Design review of the part built by this model. Coordinates are the model's own, in mm. Give positions to 0.01 mm unless a question says otherwise; leave off trailing zeros. Loops run counter-clockwise (first coordinate to the right, second up) from the corner with the lowest first, then second, coordinate; pieces in that order, holes last. Notation, with made-up numbers: (86.25, -24) - (106.25, -24) arc R11 ccw to (106.25, -6) - close; hole circle Ø11 at (-16.75, 32.25). An arc over 180 degrees is marked (long way). Write each question's results on one line, items separated by ' | '.
```python
from build123d import *

# Parameters (mm, degrees)
SKETCH1_W           = 279.4
SKETCH1_H           = 311.15
SKETCH1_W_2         = 114.3
SKETCH1_H_2         = 12.7
SKETCH1_W_3         = 12.7
SKETCH1_H_3         = 114.3
BOSS_EXTRUDE1_DEPTH = 3.3528
SKETCH2_R           = 9.525
CUT_EXTRUDE1_DEPTH  = 6.7056


with BuildPart() as part:
    # Sketch1 → Boss-Extrude1 (new body)
    with BuildSketch(Plane.XY):
        Rectangle(SKETCH1_W, SKETCH1_H)
        with Locations((-73.025, -161.925)):
            Rectangle(SKETCH1_W_2, SKETCH1_H_2)
        with Locations((73.025, -161.925)):
            Rectangle(SKETCH1_W_2, SKETCH1_H_2)
        with Locations((-146.05, -70.64375)):
            Rectangle(SKETCH1_W_3, SKETCH1_H_3)
        with Locations((-146.05, 70.64375)):
            Rectangle(SKETCH1_W_3, SKETCH1_H_3)
        with Locations((73.025, 161.925)):
            Rectangle(SKETCH1_W_2, SKETCH1_H_2)
        with Locations((-73.025, 161.925)):
            Rectangle(SKETCH1_W_2, SKETCH1_H_2)
    extrude(amount=BOSS_EXTRUDE1_DEPTH)

    # Sketch2 → Cut-Extrude1 (cut)
    with BuildSketch(Plane.XY.offset(3.3528)):
        with Locations((117.475, 69.85)):
            Circle(SKETCH2_R)
        with Locations((117.475, -69.85)):
            Circle(SKETCH2_R)
    extrude(amount=-CUT_EXTRUDE1_DEPTH, mode=Mode.SUBTRACT)


solid = part.part
```
Item 1: Wall thickness on probe 1 along Y at (x, z) = (118, 2.05) (3 decimals): over which ranges is the line inside the solid? List them lowest first.
Output values:
probe 1: y = -168.275 to -79.361, -60.339 to 60.339, 79.361 to 168.275
Item 2: We need section A-A on y = 69.85. Give the boundary of the cut face in (x, z), then the cut area to 3 significant figures.
Output values:
outline: (-152.4, 0) - (107.95, 0) - (107.95, 3.35) - (-152.4, 3.35) - close; (127, 0) - (139.7, 0) - (139.7, 3.35) - (127, 3.35) - close | area: 915 mm²
Item 3: We need section D-D on y = -142. Give the boundary of the cut face in (x, z).
Output values:
outline: (-139.7, 0) - (139.7, 0) - (139.7, 3.35) - (-139.7, 3.35) - close
Item 4: We need section B-B on z = 2.7. Give the number of separate pieces and of enclosed holes in the cut face, then the cut area to 3 significant figures.
Output values:
separate pieces: 1 | enclosed holes: 2 | area: 95,100 mm²
Item 5: Clearance check with flat-ended pins moving along their axes: P1, Ø1.7, axis at y = 137.5, z = 1.5, coming from the -X side; P2, Ø1, axis at y = -161.5, z = 1, coming from the -X side (3 decimals); P3, Ø1, axis at y = 163, z = 2.5, coming from the +X side (3 decimals). State where each tip first meets the part, or that it passes through.
Output values:
P1: stops at x = -139.7 | P2: stops at x = -130.175 | P3: stops at x = 130.175
Item 6: We need section C-C on x = 8. Give the boundary of the cut face in (y, z) (3 decimals), then the cut area to 3 significant figures.
Output values:
outline: (-155.575, 0) - (155.575, 0) - (155.575, 3.353) - (-155.575, 3.353) - close | area: 1,040 mm²
Item 7: Draft analysis for pull direction X (two halves, no side actions). For faces 1 (the face through (-8, 2, 0)), 2 (the face through (109.92, -75.65, 1.7)), state which applies: +X half, -X half, draft (parallel to the pull), parting line (faces both ways), or undercut.
Output values:
face 1: draft | face 2: undercut
